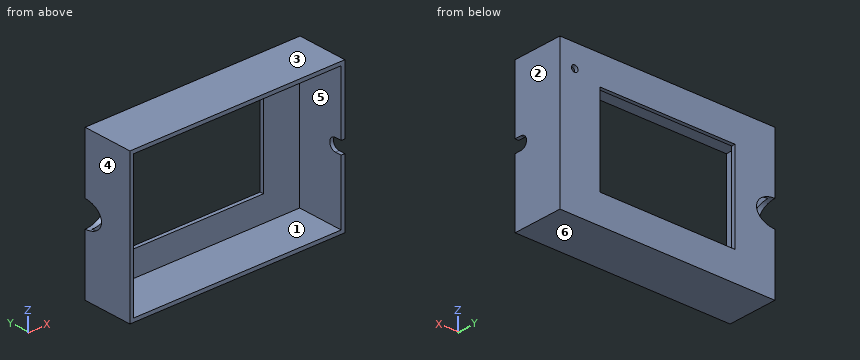
from build123d import *

# Parameters (mm, degrees)
SKETCH1_W           = 116
SKETCH1_H           = 79
SKETCH1_W_2         = 112
SKETCH1_H_2         = 75
BOSS_EXTRUDE1_DEPTH = 25
SKETCH2_W           = 116
SKETCH2_H           = 79
BOSS_EXTRUDE2_DEPTH = 2
SKETCH3_W           = 73
SKETCH3_H           = 48
CUT_EXTRUDE1_DEPTH  = 2
SKETCH4_R           = 1.75
CUT_EXTRUDE2_DEPTH  = 2
SKETCH6_R           = 7
CUT_EXTRUDE3_DEPTH  = 10
CUT_EXTRUDE4_DEPTH  = 2


with BuildPart() as part:
    # Sketch1 → Boss-Extrude1 (new body)
    with BuildSketch(Plane(origin=(0, 0, 0), x_dir=(1, 0, 0), z_dir=(0, 1, 0))):
        Rectangle(SKETCH1_W, SKETCH1_H)
        Rectangle(SKETCH1_W_2, SKETCH1_H_2, mode=Mode.SUBTRACT)
    extrude(amount=BOSS_EXTRUDE1_DEPTH)

    # Sketch2 → Boss-Extrude2 (add)
    with BuildSketch(Plane(origin=(0, 25, 0), x_dir=(1, 0, 0), z_dir=(0, 1, 0))):
        Rectangle(SKETCH2_W, SKETCH2_H)
    extrude(amount=BOSS_EXTRUDE2_DEPTH)

    # Sketch3 → Cut-Extrude1 (cut)
    with BuildSketch(Plane(origin=(0, 27, 0), x_dir=(1, 0, 0), z_dir=(0, 1, 0))):
        Rectangle(SKETCH3_W, SKETCH3_H)
    extrude(amount=-CUT_EXTRUDE1_DEPTH, mode=Mode.SUBTRACT)

    # Sketch4 → Cut-Extrude2 (cut)
    with BuildSketch(Plane(origin=(0, 27, 0), x_dir=(1, 0, 0), z_dir=(0, 1, 0))):
        with Locations((50, -27.5)):
            Circle(SKETCH4_R)
    extrude(amount=-CUT_EXTRUDE2_DEPTH, mode=Mode.SUBTRACT)

    # Sketch6 → Cut-Extrude3 (cut)
    with BuildSketch(Plane(origin=(-42.5, 42.5, 0), x_dir=(-0.707106781, -0.707106781, 0), z_dir=(0.707106781, -0.707106781, 0))):
        with Locations((21.920310217, 0)):
            Circle(SKETCH6_R)
    extrude(amount=CUT_EXTRUDE3_DEPTH, mode=Mode.SUBTRACT)

    # Sketch7 → Cut-Extrude4 (cut)
    with BuildSketch(Plane(origin=(58, 0, 0), x_dir=(0, 0, -1), z_dir=(1, 0, 0))):
        with BuildLine():
            Line((-3.375, 3.5), (-3.375, 0))
            Line((-3.375, 0), (3.375, 0))
            Line((3.375, 0), (3.375, 3.5))
            ThreePointArc((3.375, 3.5), (0, 6.875), (-3.375, 3.5))
        make_face()
    extrude(amount=-CUT_EXTRUDE4_DEPTH, mode=Mode.SUBTRACT)


solid = part.part
Work out the finished part from the listing and answer in its coordinate system (mm). Face numbers are marked on the shaded views. A direction names the side the tool comes from. Give positions to 0.01 mm unless a question says otherwise; leave off trailing zeros. Order: outer loops, then holes, each group sorted by start corner. A loop starts at its lowest first (then second) coordinate and runs counter-clockwise, first axis right, second up. Notation, with made-up numbers: M -40,7 L -9,7 A17 cw -9,37 Z; hole C -39.5,20 d1. An arc over 180 degrees is marked long. Return JSON: item names as keys, results as strings.
Q1. Find section A-A, the plane x = 50. Write down the section's boundary in (y, z), and give its area (3 significant figures).
Answer below:
{"outline": "M 0,-39.5 L 27,-39.5 L 27,25.75 L 25,25.75 L 25,-37.5 L 0,-37.5 Z; M 0,37.5 L 25,37.5 L 25,29.25 L 27,29.25 L 27,39.5 L 0,39.5 Z", "area": "251 mm^2"}
Q2. Find the intervals of material crossed by line 1 along X through (y, z) = (26.1, 27.5); line 2 along Z through (x, y) = (50, 25.5); line 3 along X through (y, z) = (4.5, 6.5), in increasing order. Write a range as [from, to].
Answer below:
{"line 1": "x = [-58, 48.25], [51.75, 58]", "line 2": "z = [-39.5, 25.75], [29.25, 39.5]", "line 3": "x = [-58, -56], [56, 58]"}
Q3. Find section B-B, the plane z = 10.5. Write down the section's boundary in (x, y).
Answer below:
{"outline": "M -58,0 L -56,0 L -56,25 L -36.5,25 L -36.5,27 L -58,27 Z; M 36.5,25 L 56,25 L 56,0 L 58,0 L 58,27 L 36.5,27 Z"}
Q4. The mould has two halves that part along Z. Classify the marked faces 3, 4, 5 and 6: pulls with the +Z half, pulls with the -Z half, needs draft (parallel to the pull), parting line crosses it, or undercut.
Answer below:
{"face 3": "pulls with the +Z half", "face 4": "needs draft", "face 5": "undercut", "face 6": "pulls with the -Z half"}
Q5. Find section C-C, the plane z = 0. Write down the section's boundary in (x, y) (1 decimal), and give its area (3 significant figures).
Answer below:
{"outline": "M -58,0 L -56,0 L -56,15.1 L -58,17.1 Z; M -48.1,27 L -46.1,25 L -36.5,25 L -36.5,27 Z; M 36.5,25 L 56,25 L 56,6.9 L 58,6.9 L 58,27 L 36.5,27 Z", "area": "133 mm^2"}
Q6. Which of the six approach directions +Z, -Z, +X, -X, +Y, -Y give full straight-line access (tool end or side, diameter ignored) to the marked faces 1 and 2?
Answer below:
{"face 1": "-Y", "face 2": "+Z, -Z, +X, +Y, -Y"}
Q7. Each of these flat-tipped pins is pushed along its axis until it touches: pin 1 (12 mm diameter, centred on x = -35.5, z = 18, fed in from -Y); pin 2 (2 mm diameter, centred on y = 25.5, z = 0.5, fed in from -X); pin 3 (3 mm diameter, centred on x = 50, z = 27.5, fed in from -Y). Where does it stop, or does it pass through?
Answer below:
{"pin 1": "stops at y = 25", "pin 2": "stops at x = -47.63", "pin 3": "passes through"}
Q8. Find section D-D, the plane z = -29. Write down the section's boundary in (x, y), and give its area (3 significant figures).
Answer below:
{"outline": "M -58,0 L -56,0 L -56,25 L 56,25 L 56,0 L 58,0 L 58,27 L -58,27 Z", "area": "332 mm^2"}
